from build123d import *

# Parameters (mm, degrees)
SKETCH1_W           = 150
SKETCH1_H           = 85
SKETCH1_R           = 2.65
BOSS_EXTRUDE1_DEPTH = 5
CUT_EXTRUDE1_DEPTH  = 5
BOSS_EXTRUDE2_START = 5
SKETCH3_R           = 2.5
SKETCH3_R_2         = 1.6
BOSS_EXTRUDE2_DEPTH = 5
SKETCH4_R           = 3
CUT_EXTRUDE2_DEPTH  = 3.2


with BuildPart() as part:
    # Sketch1 → Boss-Extrude1 (new body)
    with BuildSketch(Plane.XY):
        with Locations((75, 42.5)):
            Rectangle(SKETCH1_W, SKETCH1_H)
        with Locations((37.5, 10)):
            Circle(SKETCH1_R, mode=Mode.SUBTRACT)
        with Locations((112.5, 10)):
            Circle(SKETCH1_R, mode=Mode.SUBTRACT)
    extrude(amount=BOSS_EXTRUDE1_DEPTH)

    # Sketch2 → Cut-Extrude1 (cut)
    with BuildSketch(Plane.XY.offset(5)):
        with BuildLine():
            Line((27.4544, 72.4762), (27.4544, 70.8762))
            Line((27.4544, 70.8762), (25.8544, 70.8762))
            ThreePointArc((25.8544, 70.8762), (27.4544, 69.2762), (29.0544, 70.8762))
            ThreePointArc((29.0544, 70.8762), (28.58577085, 72.00757085), (27.4544, 72.4762))
        make_face()
        with BuildLine():
            Line((25.8544, 70.8762), (27.4544, 70.8762))
            Line((27.4544, 70.8762), (27.4544, 72.4762))
            ThreePointArc((27.4544, 72.4762), (26.32302915, 72.00757085), (25.8544, 70.8762))
        make_face()
        with BuildLine():
            Line((27.4544, 72.4762), (27.4544, 70.8762))
            Line((27.4544, 70.8762), (25.8544, 70.8762))
            ThreePointArc((25.8544, 70.8762), (27.4544, 69.2762), (29.0544, 70.8762))
            ThreePointArc((29.0544, 70.8762), (28.58577085, 72.00757085), (27.4544, 72.4762))
        make_face()
        with BuildLine():
            Line((25.8544, 70.8762), (27.4544, 70.8762))
            Line((27.4544, 70.8762), (27.4544, 72.4762))
            ThreePointArc((27.4544, 72.4762), (26.32302915, 72.00757085), (25.8544, 70.8762))
        make_face()
        with BuildLine():
            ThreePointArc((111.149409347, 22.54), (108.418038497, 23.67137085), (109.549409347, 20.94))
            Line((109.549409347, 20.94), (109.549409347, 22.54))
            Line((109.549409347, 22.54), (111.149409347, 22.54))
        make_face()
        with BuildLine():
            Line((109.549409347, 22.54), (109.549409347, 20.94))
            ThreePointArc((109.549409347, 20.94), (110.680780197, 21.40862915), (111.149409347, 22.54))
            Line((111.149409347, 22.54), (109.549409347, 22.54))
        make_face()
        with BuildLine():
            ThreePointArc((111.149409347, 22.54), (108.418038497, 23.67137085), (109.549409347, 20.94))
            Line((109.549409347, 20.94), (109.549409347, 22.54))
            Line((109.549409347, 22.54), (111.149409347, 22.54))
        make_face()
        with BuildLine():
            Line((109.549409347, 22.54), (109.549409347, 20.94))
            ThreePointArc((109.549409347, 20.94), (110.680780197, 21.40862915), (111.149409347, 22.54))
            Line((111.149409347, 22.54), (109.549409347, 22.54))
        make_face()
    extrude(amount=-CUT_EXTRUDE1_DEPTH, mode=Mode.SUBTRACT)

    # Sketch3 → Boss-Extrude2 (add)
    # profile 1 of 2: a face of its own
    with BuildSketch(Plane.XY.offset(5).offset(BOSS_EXTRUDE2_START)):
        with Locations((27.4544, 70.8762)):
            Circle(SKETCH3_R)
        with Locations((27.4544, 70.8762)):
            Circle(SKETCH3_R_2, mode=Mode.SUBTRACT)
    # profile 2 of 2: a face of its own
    with BuildSketch(Plane.XY.offset(5).offset(BOSS_EXTRUDE2_START)):
        with Locations((109.549409347, 22.54)):
            Circle(SKETCH3_R)
        with Locations((109.549409347, 22.54)):
            Circle(SKETCH3_R_2, mode=Mode.SUBTRACT)
    extrude(amount=-BOSS_EXTRUDE2_DEPTH)

    # Sketch4 → Cut-Extrude2 (cut)
    with BuildSketch(Plane(origin=(0, 0, 0), x_dir=(-1, 0, 0), z_dir=(0, 0, -1))):
        with Locations((-27.4544, 70.8762)):
            Circle(SKETCH4_R)
        with Locations((-109.549409347, 22.54)):
            Circle(SKETCH4_R)
    extrude(amount=-CUT_EXTRUDE2_DEPTH, mode=Mode.SUBTRACT)


solid = part.part
Design review of the part built by this model. Coordinates are the model's own, in mm. A direction names the side the tool comes from. Give positions to 0.01 mm unless a question says otherwise; leave off trailing zeros. Write each loop counter-clockwise with the first axis right and the second up, starting at its lowest first coordinate (ties: lowest second). Pieces come first, ordered by that corner, then holes. Notation, with made-up numbers: M 12,77 L 39,77 A21 cw 39,94 Z; hole C 20,11 d7. An arc over 180 degrees is marked long. Answer as a JSON object with one key per item and string values. Group by question number.
1) We need section A-A (x = 37.5). Give the boundary of the cut face in (y, z).
2) Clearance check with flat-ended pins moving along their axes: pin 1 Ø7 at (x, y) = (109.55, 22.54) entering from -Z; pin 2 Ø1.8 at (x, y) = (109, 22.5) entering from -Z; pin 3 Ø7 at (x, y) = (37.5, 10) entering from +Z. State where each tip first meets the part, or that it passes through.
3) Mouldability with a two-part tool opening along Y and no side actions: class faces 1 (the face through (108, 24, 10)), 2 (the face through (74, 0, 2)), 3 (the face through (108, 21, 3.2)) as released by +Y, released by -Y, zero draft, split by the parting line, or undercut.
4) For line 1 along Y through (x, z) = (37.5, 1.65); line 2 along Z through (x, y) = (95.5, 56.5); line 3 along X through (y, z) = (11, 4.5), list the stretches that pass through material, from the lowest coordinate up.
5) We need section B-B (y = 10). Give the boundary of the cut face in (x, z), and give its area (3 significant figures).
6) Tool access review of faces 4 (the face through (26.912, 68.436, 7.535)), 5 (the face through (150, 42, 2)), 6 (the face through (26.1, 68.2, 1.6)): name each direction out of +Z, -Z, +X, -X, +Y, -Y from which nothing blocks a thin tool from reaching the whole face with its end or side.
7) We need section C-C (y = 41.5). Give the boundary of the cut face in (x, z), and give its area (3 significant figures).
Answer key:
{
 "1": {"outline": "M 0,0 L 7.35,0 L 7.35,5 L 0,5 Z; M 12.65,0 L 85,0 L 85,5 L 12.65,5 Z"},
 "2": {"pin 1": "stops at z = 0", "pin 2": "passes through", "pin 3": "stops at z = 5"},
 "3": {"face 1": "zero draft", "face 2": "released by -Y", "face 3": "undercut"},
 "4": {"line 1": "y = 0 to 7.35, 12.65 to 85", "line 2": "z = 0 to 5", "line 3": "x = 0 to 35.05, 39.95 to 110.05, 114.95 to 150"},
 "5": {"outline": "M 0,0 L 34.85,0 L 34.85,5 L 0,5 Z; M 40.15,0 L 109.85,0 L 109.85,5 L 40.15,5 Z; M 115.15,0 L 150,0 L 150,5 L 115.15,5 Z", "area": "697 mm²"},
 "6": {"face 4": "+Z", "face 5": "+Z, -Z, +X, +Y, -Y", "face 6": "-Z"},
 "7": {"outline": "M 0,0 L 150,0 L 150,5 L 0,5 Z", "area": "750 mm²"}
}
